Input: dimensioned drawing with shaded views. Units: mm. Origin: part minimum x, y, z. A direction names the side the tool comes from. Give positions to 0.01 mm unless a question says otherwise; leave off trailing zeros. Write each loop counter-clockwise with the first axis right and the second up, starting at its lowest first coordinate (ties: lowest second). Pieces come first, ordered by that corner, then holes. Notation, with made-up numbers: M 74,29 L 106,29 A26 cw 106,49 Z; hole C -26,67.5 d9. An arc over 180 degrees is marked long. Use CSV: the item, a comma, the result in double quotes. Start each with the question number.
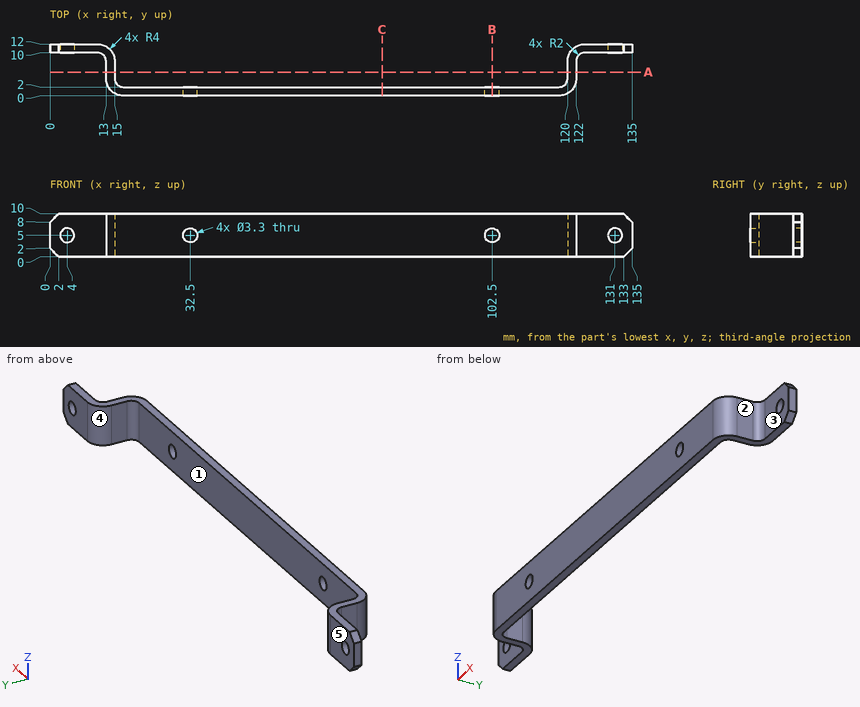
Item 1: Section A-A (y = 5.5). Return the cut outline in (x, z), plus the area to 3 significant figures.
Item 2: Set-up query: the marked faces 4 and 5. Return all of +Z, -Z, +X, -X, +Y, -Y with unobstructed straight access to the full face (end or side cutting, diameter ignored); none if empty.
Item 3: Pull-direction query (X, two-part tool) for the marked faces 1, 2 and 3; classes: released by +X, released by -X, zero draft, split by the parting line, or undercut.
Item 4: Section C-C (x = 77). Return the cut outline in (y, z).
Item 5: Material intervals for probe 1 along Z at (x, y) = (4, 11); probe 2 along X at (y, z) = (4.5, 9.25); probe 3 along Y at (x, z) = (95.5, 3), sorted ascending.
Item 6: Section B-B (x = 102.5). Return the cut outline in (y, z).
Item 7: Contact query for flat-ended pins moving along their axis: pin 1 Ø2 at (y, z) = (5.5, 6.5) entering from +X; pin 2 Ø5 at (x, z) = (128, 6.5) entering from -Y; pin 3 Ø2 at (y, z) = (7, 6) entering from -X; pin 4 Ø2 at (x, z) = (4, 5) entering from +Y. Output: stop coordinate, or through.
Output values:
1,outline,"M 13,0 L 15,0 L 15,10 L 13,10 Z; M 120,0 L 122,0 L 122,10 L 120,10 Z"
1,area,"40.0 mm2"
2,face 4,"+Z, -Z, +Y"
2,face 5,"+Z, -Z, +X, -X, +Y"
3,face 1,"undercut"
3,face 2,"released by +X"
3,face 3,"zero draft"
4,outline,"M 0,0 L 2,0 L 2,10 L 0,10 Z"
5,probe 1,"z = 0 to 3.35, 6.65 to 10"
5,probe 2,"x = 13 to 15, 120 to 122"
5,probe 3,"y = 0 to 2"
6,outline,"M 0,0 L 2,0 L 2,3.35 L 0,3.35 Z; M 0,6.65 L 2,6.65 L 2,10 L 0,10 Z"
7,pin 1,"stops at x = 122"
7,pin 2,"stops at y = 10"
7,pin 3,"stops at x = 13"
7,pin 4,"passes through"
